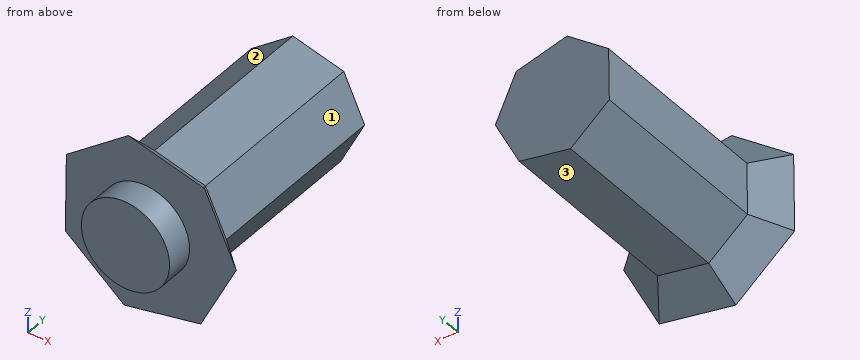
```python
from build123d import *

# Parameters (mm, degrees)
F1_DEPTH  = 103.7
F2_R      = 24.5940307027
F3_DEPTH  = 30
F1_FACE_R = 24.5940307027
F4_DEPTH  = 15
F4_TAPER  = -45


with BuildPart() as f1:
    # F0 (on Front) → F1 (new body)
    with BuildSketch(Plane.XZ):
        Polygon((22.3202445945, 25.194608101), (-6.0597066768, 32.0796431042), (-29.137253995, 14.1840528394), (-29.5342159325, -14.9930742126), (-7.9341934053, -32.7045573648), (20.6225638938, -26.5941601835), (33.9587605911, 0.1614082956), align=None)
    extrude(amount=F1_DEPTH)

    # F2 (on face) → F3 (join)
    with BuildSketch(Plane.XZ.offset(103.7)):
        Circle(F2_R)
    extrude(amount=F3_DEPTH)

    # F1_face (on face) → F4 (join)
    with BuildSketch(Plane(origin=(0.6027987413, -103.7, -0.3810429476), x_dir=(1, 0, 0), z_dir=(0, -1, 0))):
        Polygon((21.7174458532, 25.5756510486), (-6.662505418, 32.4606860518), (-29.7400527363, 14.565095787), (-30.1370146738, -14.612031265), (-8.5369921466, -32.3235144172), (20.0197651525, -26.2131172359), (33.3559618499, 0.5424512432), align=None)
        with Locations((-0.6027987413, 0.3810429476)):
            Circle(F1_FACE_R, mode=Mode.SUBTRACT)
    extrude(amount=F4_DEPTH, taper=F4_TAPER)


solid = f1.part
```
Check sheet for the modelled part. Datum: model origin and axes. Units: mm. Face numbers are marked on the shaded views. A direction names the side the tool comes from. Give positions to 0.01 mm unless a question says otherwise; leave off trailing zeros. Order: outer loops, then holes, each group sorted by start corner. A loop starts at its lowest first (then second) coordinate and runs counter-clockwise, first axis right, second up. Notation, with made-up numbers: M 0,43.5 L 44,43.5 A20 ccw 44,77.5 Z; hole C 49.25,34 d11. An arc over 180 degrees is marked long. Answer in a Markdown table with one row per item. Add a question column.
Q1. Sectioned sample at A-A, the plane y = -17. Record the boundary of the cut face in (x, z).
Q2. Gauge pin test, flat ends, axial feed: pin 1 Ø5 at (x, z) = (-23.5, -30) entering from -Y; pin 2 Ø12 at (x, y) = (34, -80) entering from -Z; pin 3 Ø4 at (y, z) = (-24, -1) entering from +X; pin 4 Ø2 at (x, z) = (37.5, -30) entering from -Y. Record the tip position at first contact, or that the pin passes through.
Q3. Thickness scan on L1, parallel to Y at x = -28.5, z = -15; L2, parallel to Z at x = 22.5, y = -72.5; L3, parallel to Z at x = -18.5, y = -90.5. Record the ranges inside material, lowest first.
Q4. Access from +Z, -Z, +X, -X, +Y, -Y to the whole of each face (thin tool, end or side, straight path). Record for the marked faces 1, 2 and 3.
Verdict:
| question | item | result |
|---|---|---|
| 1 | outline | M -29.53,-14.99 L -7.93,-32.7 L 20.62,-26.59 L 33.96,0.16 L 22.32,25.19 L -6.06,32.08 L -29.14,14.18 Z |
| 2 | pin 1 | y = -118.7 |
| 2 | pin 2 | z = -11.79 |
| 2 | pin 3 | x = 33.96 |
| 2 | pin 4 | through |
| 3 | L1 | -118.7 to 0 |
| 3 | L2 | -22.83 to 24.81 |
| 3 | L3 | -24.04 to 22.43 |
| 4 | face 1 | +Z, +X, +Y |
| 4 | face 2 | +Z, -X, +Y |
| 4 | face 3 | -Z, +X, +Y |
